Source: CAD feature listing. Evaluate the final solid. Frame: model axes, mm. Face numbers are marked on the shaded views. A direction names the side the tool comes from. Coordinates: 2 decimals unless noted, no trailing zeros. Write each loop counter-clockwise with the first axis right and the second up, starting at its lowest first coordinate (ties: lowest second). Pieces come first, ordered by that corner, then holes. Notation, with made-up numbers: (16, 75.25) - (67, 75.25) arc R15 ccw to (67, 100.25) - close; hole circle Ø4 at (-26.75, 72). An arc over 180 degrees is marked (long way). One line per item, written item: value.
from build123d import *

# Parameters (mm, degrees)
SKETCH1_W            = 35
SKETCH1_H            = 105
BOSS_EXTRUDE1_DEPTH  = 6
M4_CLEARANCE_HOLE1_D = 4.8
LPATTERN2_COUNT      = 2
LPATTERN2_PITCH      = 10
SKETCH5_W            = 4.8
SKETCH5_H            = 10
SKETCH5_W_2          = 4.730666207
SKETCH5_H_2          = 10.572708501
CUT_EXTRUDE1_DEPTH   = 88.085432636
SKETCH6_W            = 18.2
SKETCH6_H            = 18.2
CUT_EXTRUDE2_DEPTH   = 4
SKETCH7_W            = 7
SKETCH7_H            = 7
CUT_EXTRUDE3_DEPTH   = 87.970527062
SKETCH8_W            = 6
SKETCH8_H            = 23.2
CUT_EXTRUDE4_DEPTH   = 4
FILLET1_R            = 10
CUT_EXTRUDE5_START   = -6
SKETCH9_W            = 37.049954943
SKETCH9_H            = 47.5
CUT_EXTRUDE5_DEPTH   = 3
FILLET2_R            = 30
FILLET3_R            = 30
FILLET4_R            = 1
SKETCH14_W           = 7
SKETCH14_H           = 2
BOSS_EXTRUDE2_DEPTH  = 7
SKETCH16_W           = 7
SKETCH16_H           = 7
CUT_EXTRUDE6_DEPTH   = 10


with BuildPart() as part:
    # Sketch1 → Boss-Extrude1 (new body)
    with BuildSketch(Plane(origin=(0, 0, 0), x_dir=(1, 0, 0), z_dir=(0, 1, 0))):
        with Locations((0.111940299, -32.574626866)):
            Rectangle(SKETCH1_W, SKETCH1_H)
    extrude(amount=BOSS_EXTRUDE1_DEPTH)

    # M4 Clearance Hole1 (through all)
    with Locations(Plane(origin=(0, 6, 0), x_dir=(1, 0, 0), z_dir=(0, 1, 0))):
        with Locations((-12.388059701, 14.925373134), (12.611940299, 14.925373134), (12.611940299, -10.074626866), (-12.388059701, -10.074626866)):
            m4_clearance_hole1 = Hole(M4_CLEARANCE_HOLE1_D / 2)

    # LPattern2: M4 Clearance Hole1 ×2
    with Locations(*[(0, 0, i * LPATTERN2_PITCH) for i in range(1, LPATTERN2_COUNT)]):
        add(m4_clearance_hole1, mode=Mode.SUBTRACT)

    # Sketch5 → Cut-Extrude1 (cut, through all)
    with BuildSketch(Plane(origin=(0, 6, 0), x_dir=(1, 0, 0), z_dir=(0, 1, 0))):
        with Locations((-12.388059701, 9.925373134)):
            Rectangle(SKETCH5_W, SKETCH5_H)
        with Locations((-12.388059701, -15.074626866)):
            Rectangle(SKETCH5_W, SKETCH5_H)
        with Locations((12.577273403, 9.639018884)):
            Rectangle(SKETCH5_W_2, SKETCH5_H_2)
        with Locations((12.577273403, -15.360981116)):
            Rectangle(SKETCH5_W_2, SKETCH5_H_2)
    extrude(amount=-CUT_EXTRUDE1_DEPTH, mode=Mode.SUBTRACT)

    # Sketch6 → Cut-Extrude2 (cut)
    with BuildSketch(Plane(origin=(0, 6, 0), x_dir=(1, 0, 0), z_dir=(0, 1, 0))):
        with Locations((0.111940299, -72.074626866)):
            Rectangle(SKETCH6_W, SKETCH6_H)
    extrude(amount=-CUT_EXTRUDE2_DEPTH, mode=Mode.SUBTRACT)

    # Sketch7 → Cut-Extrude3 (cut, through all)
    with BuildSketch(Plane(origin=(0, 2, 0), x_dir=(1, 0, 0), z_dir=(0, 1, 0))):
        with Locations((0.111940299, -72.074626866)):
            Rectangle(SKETCH7_W, SKETCH7_H)
    extrude(amount=-CUT_EXTRUDE3_DEPTH, mode=Mode.SUBTRACT)

    # Sketch8 → Cut-Extrude4 (cut)
    with BuildSketch(Plane(origin=(0, 6, 0), x_dir=(1, 0, 0), z_dir=(0, 1, 0))):
        with Locations((0.111940299, -72.074626866)):
            Rectangle(SKETCH8_W, SKETCH8_H)
    extrude(amount=-CUT_EXTRUDE4_DEPTH, mode=Mode.SUBTRACT)

    # Fillet1
    fillet1_edges = [part.edges().sort_by_distance(p)[0] for p in [
        (17.611940299, 3, 85.074626866),
        (-17.388059701, 3, 85.074626866),
    ]]
    fillet(fillet1_edges, radius=FILLET1_R)

    # Sketch9 → Cut-Extrude5 (cut)
    with BuildSketch(Plane.XZ.offset(CUT_EXTRUDE5_START)):
        with Locations((1.136917771, 61.324626866)):
            Rectangle(SKETCH9_W, SKETCH9_H)
    extrude(amount=CUT_EXTRUDE5_DEPTH, mode=Mode.SUBTRACT)

    # Fillet2
    # the kernel refuses this fillet: 30 mm, written as the material it adds along each edge
    with BuildSketch(Plane(origin=(-17.388059701, 3, 37.574626866), x_dir=(0, 1, 0), z_dir=(1, 0, 0))) as fillet2_piece_1:
        with BuildLine():
            CenterArc((30, 13.076696831), FILLET2_R, 180, 25.841932763)
            Line((0, 13.076696831), (-0.6, 13.076696831))
            Line((-0.6, 13.076696831), (-0.6, 0))
            Line((-0.6, 0), (0, -0.6))
            ThreePointArc((0, -0.6), (1.5, -0.6), (2.46, -0.261533937))
            Line((2.46, -0.261533937), (3, 0))
        make_face()
    extrude(amount=35)

    # Fillet3
    fillet3_edges = [part.edges().sort_by_distance(p)[0] for p in [
        (0.111940299, 6, 37.574626866),
    ]]
    fillet(fillet3_edges, radius=FILLET3_R)

    # Fillet4
    fillet4_edges = [part.edges().sort_by_distance(p)[0] for p in [
        (-17.388059701, 3, -19.925373134),
        (17.611940299, 3, -19.925373134),
    ]]
    fillet(fillet4_edges, radius=FILLET4_R)

    # Sketch14 → Boss-Extrude2 (add)
    with BuildSketch(Plane(origin=(-3.388059701, 0, 0), x_dir=(0, 0, -1), z_dir=(1, 0, 0))):
        with Locations((-72.074626866, 1)):
            Rectangle(SKETCH14_W, SKETCH14_H)
    extrude(amount=BOSS_EXTRUDE2_DEPTH)

    # Sketch16 → Cut-Extrude6 (cut)
    with BuildSketch(Plane(origin=(0, 3, 0), x_dir=(1, 0, 0), z_dir=(0, 1, 0))):
        with Locations((0.111940299, -75.074626866)):
            Rectangle(SKETCH16_W, SKETCH16_H)
    extrude(amount=-CUT_EXTRUDE6_DEPTH, mode=Mode.SUBTRACT)


solid = part.part
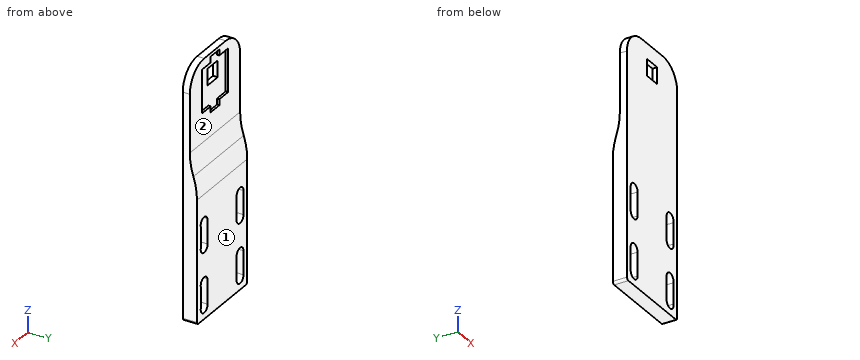
1) Section query B-B on z = -12.5. Output: boundary loops of the cut face in (x, y).
Values found:
outline: (-17.39, 0) - (-14.79, 0) - (-14.79, 6) - (-17.39, 6) - close; (-9.99, 0) - (10.21, 0) - (10.21, 6) - (-9.99, 6) - close; (14.94, 0) - (17.61, 0) - (17.61, 6) - (14.94, 6) - close
2) Section query C-C on x = 14. Output: boundary loops of the cut face in (y, z), then the cut area to 3 significant figures.
Values found:
outline: (0, -19.93) - (6, -19.93) - (6, -16.88) - (0, -16.88) - close; (0, -2.97) - (6, -2.97) - (6, 8.12) - (0, 8.12) - close; (0, 22.03) - (6, 22.03) - (6, 31.92) arc R30 ccw to (4.5, 41.28) arc R30 cw to (3, 50.65) - (3, 82.77) - (0, 82.77) - close
area: 325 mm2
3) Section query A-A on y = 1.05. State how many separate pieces and enclosed holes the cut face has, then the cut area to 3 significant figures.
Values found:
separate pieces: 1
enclosed holes: 5
area: 3,320 mm2
4) Material intervals for line 1 (X direction, y = 2.15, z = -6); line 2 (Z direction, x = 8, y = 2.55); line 3 (Y direction, x = 13.5, z = 32.5), sorted ascending.
Values found:
line 1: -17.39 to -14.79, -9.99 to 10.21, 14.94 to 17.61
line 2: -19.93 to 62.97, 81.17 to 85.07
line 3: 0 to 5.99
5) Reachability of the marked faces 1 and 2 from +Z, -Z, +X, -X, +Y, -Y: full face, straight path, thin tool, end or side. Return the list, or none.
Values found:
face 1: +Z, -Z, +X, -X, +Y
face 2: +Z, +X, -X, +Y
6) Section query D-D on x = 6.5. Output: boundary loops of the cut face in (y, z), then the cut area to 3 significant figures.
Values found:
outline: (0, -19.93) - (6, -19.93) - (6, 31.92) arc R30 ccw to (4.5, 41.28) arc R30 cw to (3, 50.65) - (3, 62.97) - (2, 62.97) - (2, 81.17) - (3, 81.17) - (3, 85.07) - (0, 85.07) - close
area: 480 mm2
7) Contact query for flat-ended pins moving along their axis: P1, Ø0.5, axis at y = 2.5, z = 82.5, coming from the +X side; P2, Ø17, axis at x = 2.5, z = 64, coming from the +Y side; P3, Ø1.1, axis at y = 2.5, z = 76, coming from the -X side; P4, Ø4, axis at x = 12.61, z = 10.07, coming from the +Y side. Output: stop coordinate, or through.
Values found:
P1: x = 14.58
P2: y = 3
P3: x = -17.38
P4: through
